Can you work these out from the drawing? Everything is in mm from the part's minimum corner. A direction names the side the tool comes from. Give positions to 0.01 mm unless a question says otherwise; leave off trailing zeros. Loops run counter-clockwise (first coordinate to the right, second up) from the corner with the lowest first, then second, coordinate; pieces in that order, holes last. Notation, with made-up numbers: (10.25, 83.5) - (26.25, 83.5) arc R21 ccw to (26.25, 103.5) - close; hole circle Ø1 at (4, -5). An arc over 180 degrees is marked (long way). Answer in a Markdown table with one row per item.
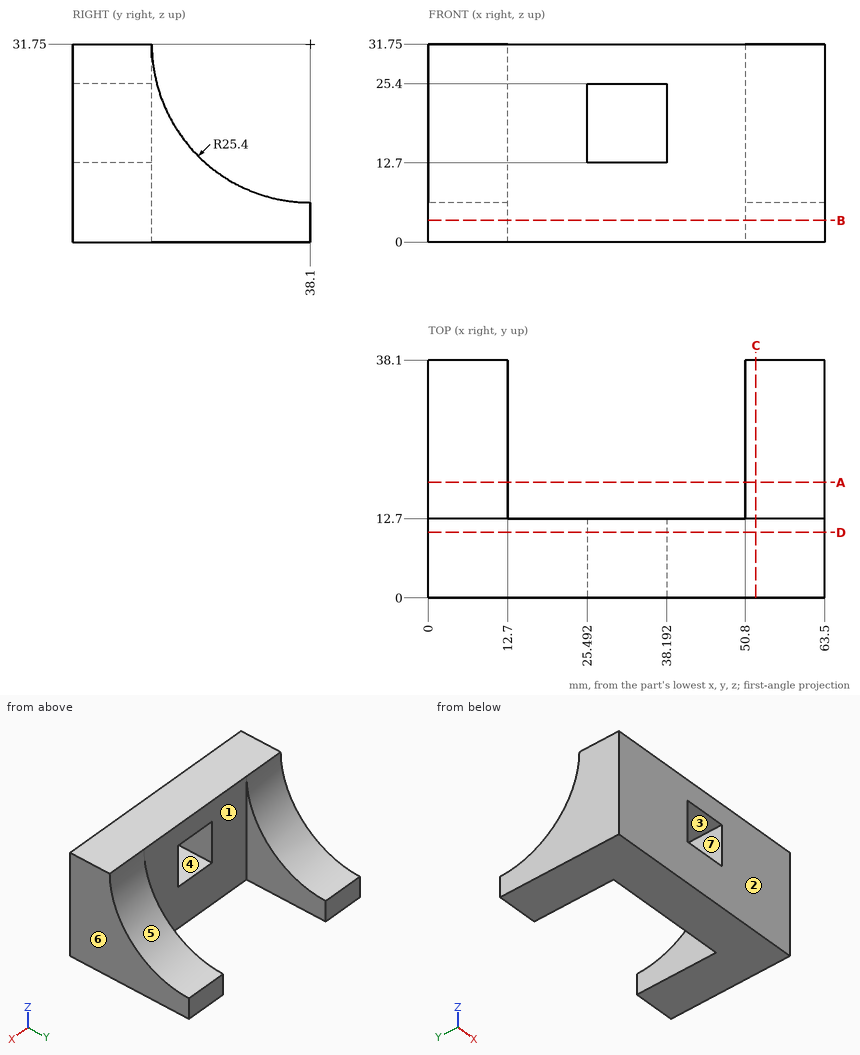
Q1. On a 3-axis mill with a long thin cutter (end or side, diameter ignored), from which of +Z, -Z, +X, -X, +Y, -Y can I reach the whole of each face in a straight line? I mean the marked faces 1, 2 and 3. Say none if no direction works.
Checked values:
| item | result |
|---|---|
| face 1 | +Z, -Z, +Y |
| face 2 | +Z, -Z, +X, -X, -Y |
| face 3 | +Y, -Y |
Q2. If I drill on line 1 (X direction, y = 20, z = 4); line 2 (Z direction, x = 33.5, y = 7); line 3 (X direction, y = 3, z = 18), over which ranges is the centre line in solid material (lowest first)? Write a range as [from, to].
Checked values:
| item | result |
|---|---|
| line 1 | x = [0, 12.7], [50.8, 63.5] |
| line 2 | z = [0, 12.7], [25.4, 31.75] |
| line 3 | x = [0, 25.49], [38.19, 63.5] |
Q3. If we mould it in two halves opening along Z, with no side actions, what happens to the marked faces 4, 5, 6 and 7? For each: released by +Z, released by -Z, zero draft, split by the parting line, or undercut.
Checked values:
| item | result |
|---|---|
| face 4 | undercut |
| face 5 | released by +Z |
| face 6 | zero draft |
| face 7 | undercut |
Q4. For pin 1 (16 mm diameter, centred on x = 29.5, z = 10.5, fed in from +Y), with a flat end and sliding along its axis, tell me the tip position at first contact or that it passes through.
Checked values:
| item | result |
|---|---|
| pin 1 | stops at y = 12.7 |
Q5. Imagine slicing it at A-A, the plane y = 18.5. Write out the boundary of the cut face in (x, z) (1 decimal), and give its area (3 significant figures).
Checked values:
| item | result |
|---|---|
| outline | (0, 0) - (12.7, 0) - (12.7, 15.6) - (0, 15.6) - close; (50.8, 0) - (63.5, 0) - (63.5, 15.6) - (50.8, 15.6) - close |
| area | 396 mm² |
Q6. Imagine slicing it at D-D, the plane y = 10.5. Write out the boundary of the cut face in (x, z), and give its area (3 significant figures).
Checked values:
| item | result |
|---|---|
| outline | (0, 0) - (63.5, 0) - (63.5, 31.75) - (0, 31.75) - close; hole (25.49, 12.7) - (38.19, 12.7) - (38.19, 25.4) - (25.49, 25.4) - close |
| area | 1,850 mm² |
Q7. Imagine slicing it at B-B, the plane z = 3.5. Write out the boundary of the cut face in (x, y), and give its area (3 significant figures).
Checked values:
| item | result |
|---|---|
| outline | (0, 0) - (63.5, 0) - (63.5, 38.1) - (50.8, 38.1) - (50.8, 12.7) - (12.7, 12.7) - (12.7, 38.1) - (0, 38.1) - close |
| area | 1,450 mm² |
Q8. Imagine slicing it at C-C, the plane x = 52.5. Write out the boundary of the cut face in (y, z), and give its area (3 significant figures).
Checked values:
| item | result |
|---|---|
| outline | (0, 0) - (38.1, 0) - (38.1, 6.35) arc R25.4 cw to (12.7, 31.75) - (0, 31.75) - close |
| area | 703 mm² |
